```python
from build123d import *

# Parameters (mm, degrees)
F1_DEPTH = 2.5
F3_DEPTH = 5.001
F4_R     = 1.25
F5_DEPTH = 5.001


with BuildPart() as f1:
    # F0 (on Top) → F1 (new body, symmetric)
    with BuildSketch(Plane.XY):
        with BuildLine():
            ThreePointArc((50, 2.5), (48.535534, 6.035534), (45, 7.5))
            Line((45, 7.5), (-45, 7.5))
            ThreePointArc((-45, 7.5), (-48.535534, 6.035534), (-50, 2.5))
            Line((-50, 2.5), (-50, -2.5))
            ThreePointArc((-50, -2.5), (-48.535534, -6.035534), (-45, -7.5))
            Line((-45, -7.5), (45, -7.5))
            ThreePointArc((45, -7.5), (48.535534, -6.035534), (50, -2.5))
            Line((50, -2.5), (50, 2.5))
        make_face()
    extrude(amount=F1_DEPTH, both=True)

    # F2 (on face) → F3 (cut, through all)
    with BuildSketch(Plane.XY.offset(2.5)):
        with BuildLine():
            Line((42.5, 2.5), (-42.5, 2.5))
            ThreePointArc((-42.5, 2.5), (-44.267767, 1.767767), (-45, 0))
            ThreePointArc((-45, 0), (-44.267767, -1.767767), (-42.5, -2.5))
            Line((-42.5, -2.5), (42.5, -2.5))
            ThreePointArc((42.5, -2.5), (44.267767, -1.767767), (45, 0))
            ThreePointArc((45, 0), (44.267767, 1.767767), (42.5, 2.5))
        make_face()
    extrude(amount=-F3_DEPTH, mode=Mode.SUBTRACT)

    # F4 (on face) → F5 (cut, through all)
    with BuildSketch(Plane.XY.offset(2.5)):
        with Locations((-47.5, 0)):
            Circle(F4_R)
    extrude(amount=-F5_DEPTH, mode=Mode.SUBTRACT)


solid = f1.part
```
The model under review builds one solid part; all positions refer to its coordinate system, in mm. A direction names the side the tool comes from. Round coordinates to 2 decimals unless told otherwise and drop trailing zeros. Order: outer loops, then holes, each group sorted by start corner. A loop starts at its lowest first (then second) coordinate and runs counter-clockwise, first axis right, second up. Notation, with made-up numbers: (-20, 69.5) -> (-14, 69.5) arc R6 ccw to (-14, 79.5) -> close; hole circle Ø7 at (66, 59.25). An arc over 180 degrees is marked (long way). Use a Markdown table: item, result.
Q1. We need section C-C on x = -47.5. Write out the cut boundary in (y, z), then the cut area to 3 significant figures.
Values:
| item | result |
|---|---|
| outline | (-6.83, -2.5) -> (-1.25, -2.5) -> (-1.25, 2.5) -> (-6.83, 2.5) -> close; (1.25, -2.5) -> (6.83, -2.5) -> (6.83, 2.5) -> (1.25, 2.5) -> close |
| area | 55.8 mm^2 |
Q2. Tool access review of faces 1 (the flat face through (-1, -2.5, 0)), 2 (the cylindrical face through (-48.57, -6, 0.04)): name each direction out of +Z, -Z, +X, -X, +Y, -Y from which nothing blocks a thin tool from reaching the whole face with its end or side.
Values:
| item | result |
|---|---|
| face 1 | +Z, -Z |
| face 2 | +Z, -Z, -X, -Y |
Q3. We need section A-A on x = 7.5. Write out the cut boundary in (y, z).
Values:
| item | result |
|---|---|
| outline | (-7.5, -2.5) -> (-2.5, -2.5) -> (-2.5, 2.5) -> (-7.5, 2.5) -> close; (2.5, -2.5) -> (7.5, -2.5) -> (7.5, 2.5) -> (2.5, 2.5) -> close |
Q4. For line 1 (Y direction, x = -27.5, z = -1.75); line 2 (X direction, y = 1, z = 0.55); line 3 (X direction, y = -0.75, z = 0.9), list the stretches that pass through material, from the lowest coordinate up.
Values:
| item | result |
|---|---|
| line 1 | y = -7.5 to -2.5, 2.5 to 7.5 |
| line 2 | x = -50 to -48.25, -46.75 to -44.79, 44.79 to 50 |
| line 3 | x = -50 to -48.5, -46.5 to -44.88, 44.88 to 50 |
Q5. Clearance check with a flat-ended pin moving along its axis: P1, Ø2, axis at x = -47.5, y = 0, coming from the +Z side. State where the tip first meets the part, or that it passes through.
Values:
| item | result |
|---|---|
| P1 | passes through |
Q6. We need section B-B on z = -1.05. Write out the cut boundary in (x, y).
Values:
| item | result |
|---|---|
| outline | (-50, -2.5) arc R5 ccw to (-45, -7.5) -> (45, -7.5) arc R5 ccw to (50, -2.5) -> (50, 2.5) arc R5 ccw to (45, 7.5) -> (-45, 7.5) arc R5 ccw to (-50, 2.5) -> close; hole circle Ø2.5 at (-47.5, 0); hole (-42.5, -2.5) -> (42.5, -2.5) arc R2.5 ccw to (42.5, 2.5) -> (-42.5, 2.5) arc R2.5 ccw to start |
Q7. Mouldability with a two-part tool opening along Y and no side actions: class faces 3 (the flat face through (-50, 0, 0)), 4 (the cylindrical face through (-48.5, 6.07, 0.04)), 5 (the flat face through (1, 2.5, 0)) as +Y half, -Y half, draft (parallel to the pull), parting line (faces both ways), or undercut.
Values:
| item | result |
|---|---|
| face 3 | draft |
| face 4 | +Y half |
| face 5 | undercut |
